```python
from build123d import *

# Parameters (mm, degrees)
F1_DEPTH = 10


with BuildPart() as f1:
    # F0 (on Top) → F1 (new body)
    with BuildSketch(Plane.XY):
        with BuildLine():
            Line((0, 25), (0, 0))
            Line((0, 0), (120, 0))
            Line((120, 0), (95, 25))
            Line((95, 25), (50, 25))
            ThreePointArc((50, 25), (30, 45), (10, 25))
            Line((10, 25), (0, 25))
        make_face()
        with BuildLine():
            ThreePointArc((20, 25), (30, 35), (40, 25))
            ThreePointArc((40, 25), (30, 15), (20, 25))
        make_face(mode=Mode.SUBTRACT)
    extrude(amount=F1_DEPTH)


solid = f1.part
```
The model under review builds one solid part; all positions refer to its coordinate system, in mm. A direction names the side the tool comes from. Round coordinates to 2 decimals unless told otherwise and drop trailing zeros. Loops run counter-clockwise (first coordinate to the right, second up) from the corner with the lowest first, then second, coordinate; pieces in that order, holes last. Notation, with made-up numbers: M -8.75,-10 L 10.25,-10 A14 cw 10.25,15 Z; hole C -36,-27.5 d10. An arc over 180 degrees is marked long. Answer as a JSON object with one key per item and string values.
(1) To check wall thickness, follow line 1 along Y through (x, z) = (30, 4); line 2 along Y through (x, z) = (67, 4); line 3 along X through (y, z) = (21.5, 6.75). State the ranges of each line that lie inside material, in increasing order.
Resolved:
{"line 1": "0 to 15, 35 to 45", "line 2": "0 to 25", "line 3": "0 to 20.63, 39.37 to 98.5"}
(2) Take a section at C-C on y = 19.5. Give the boundary of the cut face in (x, z), and give its area (3 significant figures).
Resolved:
{"outline": "M 0,0 L 21.65,0 L 21.65,10 L 0,10 Z; M 38.35,0 L 100.5,0 L 100.5,10 L 38.35,10 Z", "area": "838 mm²"}
(3) Clearance check with flat-ended pins moving along their axes: P1, Ø1.5, axis at y = 19, z = 8, coming from the +X side; P2, Ø18, axis at x = 30, y = 25, coming from the +Z side; P3, Ø5, axis at x = 62.5, z = 5.5, coming from the +Y side; P4, Ø2, axis at y = 19, z = 8.5, coming from the +X side. State where each tip first meets the part, or that it passes through.
Resolved:
{"P1": "x = 101.75", "P2": "through", "P3": "y = 25", "P4": "x = 102"}
(4) Draft analysis for pull direction X (two halves, no side actions). For faces 1 (the flat face through (108, 12, 5)), 2 (the flat face through (0, 13, 5)), 3 (the cylindrical face through (39.54, 22, 4.93)), 4 (the flat face through (5, 25, 5)), state which applies: released by +X, released by -X, zero draft, split by the parting line, or undercut.
Resolved:
{"face 1": "released by +X", "face 2": "released by -X", "face 3": "undercut", "face 4": "zero draft"}
(5) Take a section at D-D on x = 59.5. Give the boundary of the cut face in (y, z), and give its area (3 significant figures).
Resolved:
{"outline": "M 0,0 L 25,0 L 25,10 L 0,10 Z", "area": "250 mm²"}
(6) Take a section at A-A on x = 30. Give the boundary of the cut face in (y, z), and give its area (3 significant figures).
Resolved:
{"outline": "M 0,0 L 15,0 L 15,10 L 0,10 Z; M 35,0 L 45,0 L 45,10 L 35,10 Z", "area": "250 mm²"}
(7) Tool access review of faces 5 (the flat face through (46, 18, 10)), 6 (the flat face through (73, 25, 5)): name each direction out of +Z, -Z, +X, -X, +Y, -Y from which nothing blocks a thin tool from reaching the whole face with its end or side.
Resolved:
{"face 5": "+Z, +X, -X, +Y, -Y", "face 6": "+Z, -Z, +X, +Y"}
(8) Take a section at B-B on z = 7. Give the boundary of the cut face in (x, y).
Resolved:
{"outline": "M 0,0 L 120,0 L 95,25 L 50,25 A20 ccw 10,25 L 0,25 Z; hole C 30,25 d20"}
